```python
from build123d import *

# Parameters (mm, degrees)
F0_R     = 23.5
F0_R_2   = 1.651
F0_R_3   = 6.6
F1_DEPTH = 5
F2_W     = 49.363366
F2_H     = 41.91
F3_DEPTH = 5
F4_W     = 5
F4_H     = 41.91
F5_DEPTH = 40
F6_R     = 20.955
F7_DEPTH = 5
F8_R     = 1.651
F8_R_2   = 3
F9_DEPTH = 25.4
F10_SIZE = 5.08


with BuildPart() as f1:
    # F0 (on Front) → F1 (new body)
    with BuildSketch(Plane.XZ):
        Circle(F0_R)
        with Locations((8.030942, -13.91)):
            Circle(F0_R_2, mode=Mode.SUBTRACT)
        with Locations((-16.061884, 0)):
            Circle(F0_R_2, mode=Mode.SUBTRACT)
        Circle(F0_R_3, mode=Mode.SUBTRACT)
        with Locations((8.030942, 13.91)):
            Circle(F0_R_2, mode=Mode.SUBTRACT)
    extrude(amount=F1_DEPTH)

    # F2 (on Front) → F3 (join)
    with BuildSketch(Plane.XZ):
        with Locations((35.318317, 0)):
            Rectangle(F2_W, F2_H)
    extrude(amount=F3_DEPTH)

    # F4 (on face) → F5 (join)
    with BuildSketch(Plane(origin=(0, 0, 0), x_dir=(-1, 0, 0), z_dir=(0, 1, 0))):
        with Locations((-57.5, 0)):
            Rectangle(F4_W, F4_H)
    extrude(amount=F5_DEPTH)

    # F6 (on face) → F7 (join)
    with BuildSketch(Plane(origin=(55, 0, 0), x_dir=(0, -1, 0), z_dir=(-1, 0, 0))):
        with Locations((-40, 0)):
            Circle(F6_R)
    extrude(amount=-F7_DEPTH)

    # F8 (on face) → F9 (cut)
    with BuildSketch(Plane(origin=(55, 0, 0), x_dir=(0, -1, 0), z_dir=(-1, 0, 0))):
        with Locations((-40, 6.075)):
            Circle(F8_R)
        with Locations((-46.075, 0)):
            Circle(F8_R)
        with Locations((-40, -6.075)):
            Circle(F8_R)
        with Locations((-33.925, 0)):
            Circle(F8_R)
        with Locations((-40, 0)):
            Circle(F8_R_2)
    extrude(amount=-F9_DEPTH, mode=Mode.SUBTRACT)

    # F10
    f10_edges = [f1.edges().sort_by_distance(p)[0] for p in [
        (55, 0, 0),
        (60, -5, 0),
    ]]
    chamfer(f10_edges, length=F10_SIZE)


solid = f1.part
```
Model file for the job. Use its own axes, mm. A direction names the side the tool comes from. Give positions to 0.01 mm unless a question says otherwise; leave off trailing zeros. Loops run counter-clockwise (first coordinate to the right, second up) from the corner with the lowest first, then second, coordinate; pieces in that order, holes last. Notation, with made-up numbers: (-31, 23) - (20, 23) arc R9 cw to (20, 38) - close; hole circle Ø11 at (27, 73). An arc over 180 degrees is marked (long way). One line per item, written item: value. Start each with the question number.
1. Pull direction Z, two halves, no side cores. Call faces 5 (the cylindrical face through (57, 43, 0)), 6 (the cylindrical face through (-23.49, -2.46, 0.67)), 7 (the flat face through (13, 0, 0)): pulls with the +Z half, pulls with the -Z half, needs draft (parallel to the pull), parting line crosses it, or undercut.
2. Slice it at A-A (x = 0). List the corners of the cut face in (y, z), plus the area to 3 significant figures.
3. Probe L1, parallel to Z at x = 57, y = 40 (3 decimals); L2, parallel to Y at x = 46, z = -8.5; L3, parallel to X at y = 17.5, z = 17. List the from-to ranges inside material, lowest first. Write a range as from..to.
4. Slice it at C-C (z = -13.91). List the corners of the cut face in (x, y), plus the area to 3 significant figures.
5. Pin check, flat tips, straight feed: pin 1 (12.5 mm diameter, centred on y = 32.5, z = 0, fed in from -X); pin 2 (10 mm diameter, centred on x = 48.5, z = -4, fed in from +Y); pin 3 (14 mm diameter, centred on x = 14, z = 6, fed in from +Y). Stop position of each tip, or through.
6. Slice it at B-B (z = 0). List the corners of the cut face in (x, y) (3 decimals).
7. Slice it at D-D (z = 17.5). List the corners of the cut face in (x, y), plus the area to 3 significant figures.
8. Which spindle directions (+Z, -Z, +X, -X, +Y, -Y) get a long thin tool onto all of the face, cutting with end or side? Do faces 1 (the flat face through (46, -1, -20.955)), 2 (the cylindrical face through (-4.864, -2.465, 4.461)), 3 (the flat face through (46, -1, 20.955)), 4 (the flat face through (55, 26, 0)). Say none if no direction does.
Solution:
1. face 5: undercut
1. face 6: parting line crosses it
1. face 7: needs draft
2. outline: (-5, -23.5) - (0, -23.5) - (0, -6.6) - (-5, -6.6) - close; (-5, 6.6) - (0, 6.6) - (0, 23.5) - (-5, 23.5) - close
2. area: 169 mm^2
3. L1: z = -20.955..-7.726, -4.424..-3, 3..4.424, 7.726..20.955
3. L2: y = -5..0
3. L3: x = 55..60
4. outline: (-18.94, -5) - (6.38, -5) - (6.38, 0) - (-18.94, 0) - close; (9.68, -5) - (54.92, -5) - (60, 0.08) - (60, 55.67) - (55, 55.67) - (55, 5.08) - (49.92, 0) - (9.68, 0) - close
4. area: 657 mm^2
5. pin 1: stops at x = 55
5. pin 2: stops at y = 3.58
5. pin 3: stops at y = 0
6. outline: (-23.5, -5) - (-17.713, -5) - (-17.713, 0) - (-23.5, 0) - close; (-14.411, -5) - (-6.6, -5) - (-6.6, 0) - (-14.411, 0) - close; (6.6, -5) - (54.92, -5) - (60, 0.08) - (60, 32.274) - (55, 32.274) - (55, 5.08) - (49.92, 0) - (6.6, 0) - close; (55, 35.576) - (60, 35.576) - (60, 37) - (55, 37) - close; (55, 43) - (60, 43) - (60, 44.424) - (55, 44.424) - close; (55, 47.726) - (60, 47.726) - (60, 60.955) - (55, 60.955) - close
7. outline: (-15.68, -5) - (54.92, -5) - (60, 0.08) - (60, 51.53) - (55, 51.53) - (55, 5.08) - (49.92, 0) - (-15.68, 0) - close
7. area: 636 mm^2
8. face 1: -Z, +X, +Y, -Y
8. face 2: +Y, -Y
8. face 3: +Z, +X, +Y, -Y
8. face 4: +Z, -Z, -X, +Y
